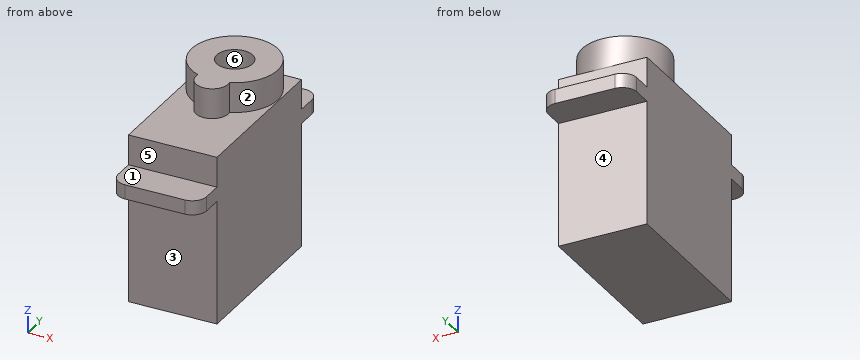
```python
from build123d import *

# Parameters (mm, degrees)
SKETCH3_W           = 22.5
SKETCH3_H           = 23.5
BOSS_EXTRUDE1_DEPTH = 6.175
SKETCH4_W           = 12.35
SKETCH4_H           = 32
BOSS_EXTRUDE2_DEPTH = 2
BOSS_EXTRUDE3_DEPTH = 4.2
SKETCH6_R           = 2.5
CUT_EXTRUDE1_DEPTH  = 4.2
FILLET1_R           = 2


with BuildPart() as part:
    # Sketch3 → Boss-Extrude1 (new body, symmetric)
    with BuildSketch(Plane(origin=(0, -28.275548605, 0), x_dir=(0, 1, 0), z_dir=(1, 0, 0))):
        with Locations((24.609729517, 167.116706922)):
            Rectangle(SKETCH3_W, SKETCH3_H)
    extrude(amount=BOSS_EXTRUDE1_DEPTH, both=True)

    # Sketch4 → Boss-Extrude2 (add)
    with BuildSketch(Plane.XY.offset(174.666706922)):
        with Locations((0, -3.665819089)):
            Rectangle(SKETCH4_W, SKETCH4_H)
    extrude(amount=-BOSS_EXTRUDE2_DEPTH)

    # Sketch5 → Boss-Extrude3 (add)
    with BuildSketch(Plane.XY.offset(178.866706922)):
        with BuildLine():
            ThreePointArc((2.210095356, -3.993944089), (0, 7.584180911), (-2.210095356, -3.993944089))
            ThreePointArc((-2.210095356, -3.993944089), (0, -6.665819089), (2.210095356, -3.993944089))
        make_face()
    extrude(amount=BOSS_EXTRUDE3_DEPTH)

    # Sketch6 → Cut-Extrude1 (cut)
    with BuildSketch(Plane.XY.offset(183.066706922)):
        with Locations((0, 1.584180911)):
            Circle(SKETCH6_R)
    extrude(amount=-CUT_EXTRUDE1_DEPTH, mode=Mode.SUBTRACT)

    # Fillet1
    fillet1_edges = [part.edges().sort_by_distance(p)[0] for p in [
        (-6.175, -19.665819089, 173.666706922),
        (6.175, 12.334180911, 173.666706922),
        (-6.175, 12.334180911, 173.666706922),
        (6.175, -19.665819089, 173.666706922),
    ]]
    fillet(fillet1_edges, radius=FILLET1_R)


solid = part.part
```
Input: part model. Units: mm. Frame: model coordinates. Face numbers are marked on the shaded views. A direction names the side the tool comes from. Coordinates: 2 decimals unless noted, no trailing zeros. Write each loop counter-clockwise with the first axis right and the second up, starting at its lowest first coordinate (ties: lowest second). Pieces come first, ordered by that corner, then holes.
1) Pin query (flat end, axial travel): pin 1 Ø2.5 at (x, y) = (0.5, 2.5) entering from +Z; pin 2 Ø1.3 at (x, z) = (0.5, 177) entering from -Y; pin 3 Ø3.5 at (x, z) = (0, 167) entering from +Y. Return the tip coordinate at first contact, or that it passes through.
2) Section D-D on y = 9. Output: boundary loops of the cut face in (x, z) (3 decimals), and give its area (3 significant figures).
3) Mould query, pull axis Y, two halves, no side actions, for the marked faces 4, 5 and 6. Classes: pulls with the +Y half, pulls with the -Y half, needs draft (parallel to the pull), parting line crosses it, or undercut.
4) Section A-A on y = -0.5. Output: boundary loops of the cut face in (x, z) (3 decimals).
5) Set-up query: the marked faces 1, 2 and 3. Return all of +Z, -Z, +X, -X, +Y, -Y with unobstructed straight access to the full face (end or side cutting, diameter ignored); none if empty.
6) Material intervals for line 1 along Y through (x, z) = (0, 182.1); line 2 along Z through (x, y) = (4.25, -17.5); line 3 along Z through (x, y) = (-1.25, -8.5), sorted ascending.
7) Section B-B on z = 177.5. Output: boundary loops of the cut face in (x, y) (3 decimals), and give its area (3 significant figures).
8) Section C-C on x = 1.25. Output: boundary loops of the cut face in (y, z), and give its area (3 significant figures).
Check result:
1. pin 1: stops at z = 178.87
1. pin 2: stops at y = -14.92
1. pin 3: stops at y = 7.58
2. outline: (-6.175, 172.667) - (6.175, 172.667) - (6.175, 174.667) - (-6.175, 174.667) - close
2. area: 24.7 mm2
3. face 4: pulls with the +Y half
3. face 5: pulls with the -Y half
3. face 6: undercut
4. outline: (-6.175, 155.367) - (6.175, 155.367) - (6.175, 178.867) - (5.626, 178.867) - (5.626, 183.067) - (1.381, 183.067) - (1.381, 178.867) - (-1.381, 178.867) - (-1.381, 183.067) - (-5.626, 183.067) - (-5.626, 178.867) - (-6.175, 178.867) - close
5. face 1: +Z, +X, -X, -Y
5. face 2: +Z
5. face 3: -Z, +X, -X, -Y
6. line 1: y = -6.67 to -0.92, 4.08 to 7.58
6. line 2: z = 172.67 to 174.67
6. line 3: z = 155.37 to 178.87
7. outline: (-6.175, -14.916) - (6.175, -14.916) - (6.175, 7.584) - (-6.175, 7.584) - close
7. area: 278 mm2
8. outline: (-19.67, 172.67) - (-14.92, 172.67) - (-14.92, 155.37) - (7.58, 155.37) - (7.58, 172.67) - (12.33, 172.67) - (12.33, 174.67) - (7.58, 174.67) - (7.58, 178.87) - (7.45, 178.87) - (7.45, 183.07) - (3.75, 183.07) - (3.75, 178.87) - (-0.58, 178.87) - (-0.58, 183.07) - (-6.29, 183.07) - (-6.29, 178.87) - (-14.92, 178.87) - (-14.92, 174.67) - (-19.67, 174.67) - close
8. area: 587 mm2
